Part model, mm, in its own coordinate system. A direction names the side the tool comes from. Give positions to 0.01 mm unless a question says otherwise; leave off trailing zeros. Write each loop counter-clockwise with the first axis right and the second up, starting at its lowest first coordinate (ties: lowest second). Pieces come first, ordered by that corner, then holes.
from build123d import *

# Parameters (mm, degrees)
F1_W     = 4
F1_H     = 2.75
F2_DEPTH = 27
F3_R     = 1.99999


# Not quite as in the source:
# - a fillet or chamfer is up to 0.001 mm smaller than in the source, because OpenCascade refuses the exact size


with BuildPart() as f2:
    # F1 (on Front) → F2 (new body)
    with BuildSketch(Plane.XZ):
        with BuildLine():
            Line((4, 16.5), (0, 16.5))
            Line((0, 16.5), (0, 5.5))
            ThreePointArc((0, 5.5), (1.0590284919, 9.8588989435), (4, 13.2459666924))
            Line((4, 13.2459666924), (4, 16.5))
        make_face()
        with BuildLine():
            ThreePointArc((1.7540333076, 0), (0.4491248054, 2.6135388083), (0, 5.5))
            Line((0, 5.5), (0, 0))
            Line((0, 0), (1.7540333076, 0))
        make_face()
        with BuildLine():
            Line((4, 5.5), (0, 5.5))
            ThreePointArc((0, 5.5), (0.4491248054, 2.6135388083), (1.7540333076, 0))
            Line((1.7540333076, 0), (4, 0))
            Line((4, 0), (4, 5.5))
        make_face()
        with BuildLine():
            ThreePointArc((4, 13.2459666924), (1.0590284919, 9.8588989435), (0, 5.5))
            Line((0, 5.5), (4, 5.5))
            Line((4, 5.5), (4, 13.2459666924))
        make_face()
        with BuildLine():
            Line((1.7540333076, 0), (0, 0))
            Line((0, 0), (0, -60.5))
            Line((0, -60.5), (4, -60.5))
            Line((4, -60.5), (4, -2.2459666924))
            ThreePointArc((4, -2.2459666924), (2.7824855787, -1.2175144213), (1.7540333076, 0))
        make_face()
        with BuildLine():
            Line((4, 0), (1.7540333076, 0))
            ThreePointArc((1.7540333076, 0), (2.7824855787, -1.2175144213), (4, -2.2459666924))
            Line((4, -2.2459666924), (4, 0))
        make_face()
        with BuildLine():
            ThreePointArc((9.5, 0), (5.6109127035, 1.6109127035), (4, 5.5))
            Line((4, 5.5), (4, 0))
            Line((4, 0), (9.5, 0))
        make_face()
        with BuildLine():
            Line((9.5, 0), (4, 0))
            Line((4, 0), (4, -2.2459666924))
            ThreePointArc((4, -2.2459666924), (11.0881382785, -3.8663128716), (17.2459666924, 0))
            Line((17.2459666924, 0), (9.5, 0))
        make_face()
        with BuildLine():
            ThreePointArc((15, 5.5), (13.3890872965, 1.6109127035), (9.5, 0))
            Line((9.5, 0), (17.2459666924, 0))
            ThreePointArc((17.2459666924, 0), (18.5508751946, 2.6135388083), (19, 5.5))
            Line((19, 5.5), (15, 5.5))
        make_face()
        with Locations((17, 6.875)):
            Rectangle(F1_W, F1_H)
    extrude(amount=F2_DEPTH)

    # F3 (radius 2 in the source; OpenCascade refuses exactly that, so slightly less here)
    f3_edges = [f2.edges().sort_by_distance(p)[0] for p in [
        (4, -27, -31.372983),
        (4, -27, 11),
        (4, 0, -31.372983),
        (4, -13.5, -60.5),
        (4, 0, 11),
        (19, -13.5, 8.25),
        (4, -13.5, 16.5),
    ]]
    fillet(f3_edges, radius=F3_R)


solid = f2.part
1) Saw through at A-A (y = -20). Write the cut outline in (x, z).
Check result:
outline: (0, -60.5) - (2, -60.5) arc R2 ccw to (4, -58.5) - (4, -2.25) arc R9.5 ccw to (19, 5.5) - (19, 6.25) arc R2 ccw to (17, 8.25) - (15, 8.25) - (15, 5.5) arc R5.5 cw to (4, 5.5) - (4, 14.5) arc R2 ccw to (2, 16.5) - (0, 16.5) - close
2) Drill centre lines: L1, parallel to X at y = -11.75, z = -56.5; L2, parallel to Z at x = 9.5, y = -12.25; L3, parallel to X at y = -12, z = -3. Where is each one in solid material? Low to high.
Check result:
L1: x = 0 to 4
L2: z = -4 to 0
L3: x = 0 to 4, 5.26 to 13.74
3) Saw through at B-B (z = -50). Write the cut outline in (x, y).
Check result:
outline: (0, -27) - (2, -27) arc R2 ccw to (4, -25) - (4, -2) arc R2 ccw to (2, 0) - (0, 0) - close
4) 3-axis set-ups, long thin cutter, end or side, ignore diameter. For faces 1 (the flat face through (16, -13, 8.25)), 2 (the cylindrical face through (15.57, -0.6, 6.86)), 3 (the cylindrical face through (15.57, -26.4, 6.86)), 4 (the flat face through (1, -13, 16.5)), 5 (the flat face through (15, -13, 7)): which of +Z, -Z, +X, -X, +Y, -Y reach the whole face in a straight line?
Check result:
face 1: +Z, +X, +Y, -Y
face 2: +Z, +Y
face 3: +Z, -Y
face 4: +Z, +X, -X, +Y, -Y
face 5: +Z, +Y, -Y
5) Mould opens along X. For faces 6 (the flat face through (4, -13, 10)), 7 (the cylindrical face through (18.43, -13.69, 7.65)), 8 (the flat face through (1.7, 0, -16.1)) say: +X half, -X half, draft (parallel to the pull), parting line (faces both ways), or undercut.
Check result:
face 6: undercut
face 7: +X half
face 8: draft
6) Flat gauge pins, fed straight in: P1, Ø7, axis at y = -10.5, z = -18, coming from the +X side; P2, Ø1.6, axis at x = 16, y = -14.5, coming from the +Z side. Where does each tip first touch, or does it go through?
Check result:
P1: stops at x = 4
P2: stops at z = 8.25
